Answer from the drawing. Dimensions are ordinates in mm from the lowest x, y and z of the part. A direction names the side the tool comes from. Give positions to 0.01 mm unless a question says otherwise; leave off trailing zeros. Loops run counter-clockwise (first coordinate to the right, second up) from the corner with the lowest first, then second, coordinate; pieces in that order, holes last. Notation, with made-up numbers: (78, -17) - (105, -17) arc R20 ccw to (105, -10) - close; hole circle Ø5 at (-11, 15.5). An arc over 180 degrees is marked (long way). Write each question's results on one line, items separated by ' | '. Start each with the question number.
Q1. For the marked faces 1 and 2, determine the directions among +Z, -Z, +X, -X, +Y, -Y from which every point of the face is accessible in a straight line to the end or side of a thin tool.
Q2. Find the intervals of material crossed by line 1 (Z direction, x = 10.4, y = 0.7); line 2 (Z direction, x = 14, y = 2.75); line 3 (Y direction, x = 9.25, z = 5), in increasing order. Write a range as from..to.
Q3. Given pin 1 (1 mm diameter, centred on y = 3.5, z = 10, fed in from -X); pin 2 (6 mm diameter, centred on x = 10, z = 7, fed in from +Y), each flat-ended and moving along its own axis, determine where each tip first touches the part or whether it passes through.
Q4. Determine the mould class of the marked faces 3, 4 and 5 for opening direction Z: +Z half, -Z half, draft (parallel to the pull), parting line (faces both ways), or undercut.
Q5. The part is cut by section C-C, the plane z = 7.5. Write down the section's boundary in (x, y), plus the area to 3 significant figures.
Q6. The part is cut by section B-B, the plane y = 9.6. Write down the section's boundary in (x, z), plus the area to 3 significant figures.
Q7. The part is cut by section D-D, the plane y = 15.25. Write down the section's boundary in (x, z).
Q8. The part is cut by section A-A, the plane x = 10.4. Write down the section's boundary in (y, z).
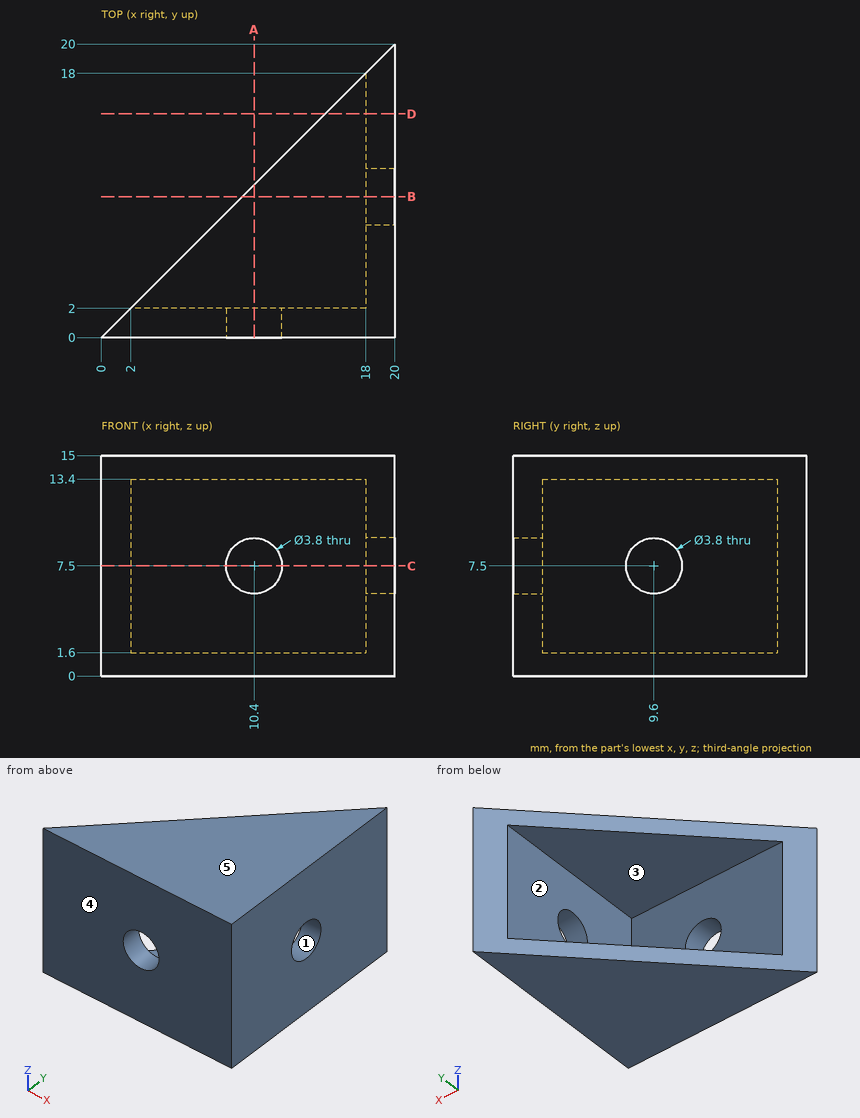
Check sheet entries:
1) face 1: +X, -X | face 2: -X, +Y
2) line 1: z = 0..5.6, 9.4..15 | line 2: z = 0..1.6, 13.4..15 | line 3: y = 0..2
3) pin 1: stops at x = 18 | pin 2: stops at y = 2
4) face 3: undercut | face 4: draft | face 5: +Z half
5) outline: (0, 0) - (8.5, 0) - (8.5, 2) - (2, 2) - close; (12.3, 0) - (20, 0) - (20, 7.7) - (18, 7.7) - (18, 2) - (12.3, 2) - close; (18, 11.5) - (20, 11.5) - (20, 20) - (18, 18) - close | area: 56.8 mm^2
6) outline: (9.6, 0) - (20, 0) - (20, 5.6) - (18, 5.6) - (18, 1.6) - (9.6, 1.6) - close; (9.6, 13.4) - (18, 13.4) - (18, 9.4) - (20, 9.4) - (20, 15) - (9.6, 15) - close | area: 49.3 mm^2
7) outline: (15.25, 0) - (20, 0) - (20, 15) - (15.25, 15) - (15.25, 13.4) - (18, 13.4) - (18, 1.6) - (15.25, 1.6) - close
8) outline: (0, 0) - (10.4, 0) - (10.4, 1.6) - (2, 1.6) - (2, 5.6) - (0, 5.6) - close; (0, 9.4) - (2, 9.4) - (2, 13.4) - (10.4, 13.4) - (10.4, 15) - (0, 15) - close
